The listing builds one solid part. Answer for the finished solid, in the listing's coordinates (mm). A direction names the side the tool comes from. Round coordinates to 2 decimals unless told otherwise and drop trailing zeros. Write each loop counter-clockwise with the first axis right and the second up, starting at its lowest first coordinate (ties: lowest second). Pieces come first, ordered by that corner, then holes.
Item 1: A tool of negligible diameter and unlimited length cuts with its end or side. For faces 1 (the face through (0, 0, -4)), 2 (the face through (0.27, 6.28, -5.92)), 3 (the face through (1.5, 7, 8)), 4 (the face through (0, 7, 4.75)), from which of +Z, -Z, +X, -X, +Y, -Y can it reach the whole face along a straight path? Write none if from no direction.
Item 2: Find section A-A on z = 0. Give the vertices of the cut face in (x, y), then the cut area to 3 significant figures.
Item 3: Find section B-B on x = 0. Give the vertices of the cut face in (y, z).
Item 4: Find section D-D on y = 7.5. Give the vertices of the cut face in (x, z).
Item 5: Find section C-C on y = 3. Give the vertices of the cut face in (x, z).
Item 6: Each of these flat-tipped pins is pushed along its axis until it touches: pin 1 (0.6 mm diameter, centred on y = 11, z = 7.5, fed in from +X); pin 2 (0.8 mm diameter, centred on x = 2.5, y = 5, fed in from -Z); pin 3 (1.5 mm diameter, centred on y = 11, z = 6, fed in from +X); pin 4 (7.5 mm diameter, centred on x = 0, z = 0, fed in from -Y). Where does it stop, or does it pass through?
Item 7: For a pull along Z with two mould halves and no side action, classify faces 5 (the face through (-1.5, 7, 8)), 6 (the face through (-5.07, 7.4, -7.13)), 7 (the face through (-3, 7, 6.62)) as +Z half, -Z half, draft (parallel to the pull), parting line (faces both ways), or undercut.
Item 8: Find the intervals of material crossed by probe 1 along X at (y, z) = (5.25, 0); probe 2 along Z at (x, y) = (-1.75, 7.5); probe 3 along Y at (x, z) = (0, -4.75), in increasing order.
```python
from build123d import *

# Parameters (mm, degrees)
SKETCH1_R           = 8.75
SKETCH1_R_2         = 3.25
BOSS_EXTRUDE1_DEPTH = 15
SKETCH2_W           = 3
SKETCH2_H           = 15
CUT_EXTRUDE2_DEPTH  = 4
SKETCH3_R           = 1.25
CUT_EXTRUDE3_DEPTH  = 8
SKETCH5_W           = 1.870469825
SKETCH5_H           = 15
CUT_EXTRUDE4_DEPTH  = 4


with BuildPart() as part:
    # Sketch1 → Boss-Extrude1 (new body)
    with BuildSketch(Plane(origin=(0, 0, 0), x_dir=(1, 0, 0), z_dir=(0, 1, 0))):
        Circle(SKETCH1_R)
        Circle(SKETCH1_R_2, mode=Mode.SUBTRACT)
    extrude(amount=BOSS_EXTRUDE1_DEPTH)

    # Sketch2 → Cut-Extrude2 (cut)
    with BuildSketch(Plane.XY.offset(8.75)):
        with Locations((0, 7.5)):
            Rectangle(SKETCH2_W, SKETCH2_H)
    extrude(amount=-CUT_EXTRUDE2_DEPTH, mode=Mode.SUBTRACT)

    # Sketch3 → Cut-Extrude3 (cut)
    with BuildSketch(Plane(origin=(0, 0, -8.75), x_dir=(-1, 0, 0), z_dir=(0, 0, -1))):
        with Locations((0, 7.5)):
            Circle(SKETCH3_R)
    extrude(amount=-CUT_EXTRUDE3_DEPTH, mode=Mode.SUBTRACT)

    # Sketch5 → Cut-Extrude4 (cut, symmetric)
    with BuildSketch(Plane.ZY):
        with Locations((5.685234913, 7.5)):
            Rectangle(SKETCH5_W, SKETCH5_H)
    extrude(amount=CUT_EXTRUDE4_DEPTH, both=True, mode=Mode.SUBTRACT)


solid = part.part
```
Check values:
1. face 1: +Z, -Z, +X, -X, -Y
1. face 2: -Z
1. face 3: +Z, +Y, -Y
1. face 4: +Y, -Y
2. outline: (-8.75, 0) - (-3.25, 0) - (-3.25, 15) - (-8.75, 15) - close; (3.25, 0) - (8.75, 0) - (8.75, 15) - (3.25, 15) - close
2. area: 165 mm2
3. outline: (0, -8.75) - (6.25, -8.75) - (6.25, -3.25) - (0, -3.25) - close; (0, 3.25) - (15, 3.25) - (15, 4.75) - (0, 4.75) - close; (8.75, -8.75) - (15, -8.75) - (15, -3.25) - (8.75, -3.25) - close
4. outline: (-4, 4.75) - (-4, 6.62) - (-1.5, 6.62) - (-1.5, 8.62) arc R8.75 ccw to (-1.25, -8.66) - (-1.25, -3) arc R3.25 cw (long way) to (1.25, -3) - (1.25, -8.66) arc R8.75 ccw to (1.5, 8.62) - (1.5, 6.62) - (4, 6.62) - (4, 4.75) - close
5. outline: (-4, 4.75) - (-4, 6.62) - (-1.5, 6.62) - (-1.5, 8.62) arc R8.75 ccw (long way) to (1.5, 8.62) - (1.5, 6.62) - (4, 6.62) - (4, 4.75) - close; hole circle Ø6.5 at (0, 0)
6. pin 1: stops at x = 4.97
6. pin 2: stops at z = -8.49
6. pin 3: stops at x = 7
6. pin 4: stops at y = 0
7. face 5: draft
7. face 6: parting line
7. face 7: undercut
8. probe 1: x = -8.75 to -3.25, 3.25 to 8.75
8. probe 2: z = -8.57 to -2.74, 2.74 to 4.75, 6.62 to 8.57
8. probe 3: y = 0 to 6.25, 8.75 to 15
